Autodesk Inventor part; units mm, degrees
ref_plane "YZ Plane" through (0, 0, 0) normal (1, 0, 0) x (0, 1, 0)
ref_plane "XZ Plane" through (0, 0, 0) normal (0, 1, 0) x (-1, 0, 0)
ref_plane "XY Plane" through (0, 0, 0) normal (0, 0, 1) x (1, 0, 0)
sketch "Sketch1" plane through (0, 0, 0) normal (1, 0, 0) x (0, 1, 0)
  arc A0 (0, -75) -> (0, 75) centre (0, 0) ccw
  line L0 (0, 75) -> (-75, 75)
  line L1 (0, -75) -> (-75, -75)
  line L2 (-75, 75) -> (-95.2073, 40)
  line L3 (-75, 75) -> (-34.5855, 75) construction
  circle A1 centre (0, 0) radius 45
  line L4 (-95.2073, 40) -> (-45.2073, 40)
  line L5 (-45.2073, 40) -> (-34.3167, 29.1095)
  line L6 (-45.2073, 40) -> (-29.8057, 40) construction
  line L7 (91.7333, 0) -> (-104.2658, 0) construction
  line L8 (-95.2073, -40) -> (-45.2073, -40)
  line L9 (-45.2073, -40) -> (-34.3167, -29.1095)
  line L10 (-45.2073, -40) -> (-29.8057, -40) construction
  line L11 (-75, -75) -> (-95.2073, -40)
  circle A2 centre (0, 0) radius 39
  line L12 (-71.5359, 69) -> (0, 69)
  arc A3 (0, -69) -> (0, 69) centre (0, 0) ccw
  line L13 (0, -69) -> (-71.5359, -69)
  line L14 (-71.5359, 69) -> (-84.815, 46)
  line L15 (-84.815, 46) -> (-39.7549, 46)
  line L16 (-39.7549, 46) -> (-29.8057, 33.7138)
  line L17 (-71.5359, -69) -> (-84.815, -46)
  line L18 (-84.815, -46) -> (-39.7549, -46)
  line L19 (-39.7549, -46) -> (-29.8057, -33.7138)
  dimension "d0" = 150
  dimension "d2" = 75
  dimension "d3" = 120
  dimension "d4" = 35
  dimension "d9" = 30
  dimension "d10" = 50
  dimension "d11" = 45
  dimension "d12" = 60
  dimension "d13" = 40
  dimension "d14" = 3.6821
  dimension "d15" = 68.5473
  dimension "d16" = 70.045
  dimension "d17" = 6
  dimension "d18" = 6
  dimension "d19" = 6
  dimension "d20" = 6
  dimension "d21" = 6
  dimension "d22" = 15.8094
extrude "Extrusion3" add sketch "Sketch1" along normal blind 50 contours L1 L11 L8 L9 A1 L19 L18 L17 L13 A3 L12 L14 L15 L16 L5 L4 L2 L0 A0
extrude "Extrusion4" add sketch "Sketch1" along normal blind 10 contours A1 | A1 L16 L15 L14 L12 A3 L13 L17 L18 L19
properties part number "Brazo 3D"
Read the model definition and answer for the solid it produces. Units are mm, in the model's axes. A direction names the side the tool comes from. Round coordinates to 2 decimals unless told otherwise and drop trailing zeros. Write each loop counter-clockwise with the first axis right and the second up, starting at its lowest first coordinate (ties: lowest second). Pieces come first, ordered by that corner, then holes. Notation, with made-up numbers: (63.5, 54.5) - (69.5, 54.5) arc R16 ccw to (69.5, 69.5) - close; hole circle Ø1 at (66.5, 39.5). An arc over 180 degrees is marked (long way). Use a Markdown table: item, result.
(1) The part is cut by section A-A (z = 0). Write down the section's boundary in (x, y), then the cut area to 3 significant figures.
Reported:
| item | result |
|---|---|
| outline | (0, -45) - (10, -45) - (10, -39) - (0, -39) - close; (0, 39) - (10, 39) - (10, 69) - (50, 69) - (50, 75) - (0, 75) - close |
| area | 660 mm2 |
(2) Each of these flat-tipped pins is pushed along its axis until it touches: pin 1 Ø12 at (x, z) = (17.5, -32.5) entering from +Y; pin 2 Ø25 at (x, y) = (29.5, -82) entering from -Z; pin 3 Ø6 at (y, z) = (46, 35) entering from +X; pin 4 Ø12 at (x, z) = (23.5, 31) entering from -Y. Where does it stop, or does it pass through?
Reported:
| item | result |
|---|---|
| pin 1 | y = 70.16 |
| pin 2 | z = -75 |
| pin 3 | x = 10 |
| pin 4 | y = -42.21 |
(3) The part is cut by section B-B (y = -56). Write down the section's boundary in (x, z), then the cut area to 3 significant figures.
Reported:
| item | result |
|---|---|
| outline | (0, -75) - (50, -75) - (50, -69) - (10, -69) - (10, -46) - (50, -46) - (50, -40) - (0, -40) - close; (0, 40) - (50, 40) - (50, 46) - (10, 46) - (10, 69) - (50, 69) - (50, 75) - (0, 75) - close |
| area | 1,660 mm2 |
(4) The part is cut by section C-C (x = 32.5). Write down the section's boundary in (y, z) (1 decimal).
Reported:
| item | result |
|---|---|
| outline | (-95.2, -40) - (-75, -75) - (0, -75) arc R75 ccw to (0, 75) - (-75, 75) - (-95.2, 40) - (-45.2, 40) - (-34.3, 29.1) arc R45 cw to (-29.8, 33.7) - (-39.8, 46) - (-84.8, 46) - (-71.5, 69) - (0, 69) arc R69 cw to (0, -69) - (-71.5, -69) - (-84.8, -46) - (-39.8, -46) - (-29.8, -33.7) arc R45 cw to (-34.3, -29.1) - (-45.2, -40) - close |
(5) The mould has two halves that part along Z. Classify faces 1 (the flat face through (24.65, -39.84, -34.63)), 2 (the flat face through (25, -37, 75)), 3 (the flat face through (50, -36, 34)), 4 (the cylindrical face through (24.65, 74.98, 1.65)): released by +Z, released by -Z, zero draft, split by the parting line, or undercut.
Reported:
| item | result |
|---|---|
| face 1 | undercut |
| face 2 | released by +Z |
| face 3 | zero draft |
| face 4 | split by the parting line |
(6) Straight lines are drawn through the part: line 1 along Z through (x, y) = (27, -70); line 2 along Z through (x, y) = (6.75, 0); line 3 along X through (y, z) = (-30, -41). For each, find the intervals that lie inside material, in ascending order. Write a range as [from, to].
Reported:
| item | result |
|---|---|
| line 1 | [-75, -69], [-46, -40], [40, 46], [69, 75] |
| line 2 | [-75, -39], [39, 75] |
| line 3 | [0, 10] |
(7) Which of the six approach directions +Z, -Z, +X, -X, +Y, -Y give full straight-line access (tool end or side, diameter ignored) to faces 5 (the cylindrical face through (4.93, -5.077, -38.668)), 6 (the flat face through (30, -63, 46)), 7 (the flat face through (24.65, -39.84, 34.63))?
Reported:
| item | result |
|---|---|
| face 5 | +X, -X |
| face 6 | +X |
| face 7 | +X, -X, -Y |
(8) The part is cut by section D-D (x = 4.5). Write down the section's boundary in (y, z), then the cut area to 3 significant figures.
Reported:
| item | result |
|---|---|
| outline | (-95.21, -40) - (-75, -75) - (0, -75) arc R75 ccw to (0, 75) - (-75, 75) - (-95.21, 40) - (-45.21, 40) - (-34.32, 29.11) arc R45 ccw to (-34.32, -29.11) - (-45.21, -40) - close; hole circle Ø78 at (0, 0) |
| area | 13,300 mm2 |
